```python
from build123d import *

# Parameters (mm, degrees)
F0_W     = 93
F0_H     = 153
F2_DEPTH = 6
F1_W     = 93
F1_H     = 14
F3_DEPTH = 2
F5_D     = 6


with BuildPart() as f2:
    # F0 (on Top) → F2 (new body)
    with BuildSketch(Plane.XY):
        with BuildLine():
            Line((-73.5, -125.5), (73.5, -125.5))
            ThreePointArc((73.5, -125.5), (79.1568542495, -123.1568542495), (81.5, -117.5))
            Line((81.5, -117.5), (81.5, 117.5))
            ThreePointArc((81.5, 117.5), (79.1568542495, 123.1568542495), (73.5, 125.5))
            Line((73.5, 125.5), (-73.5, 125.5))
            ThreePointArc((-73.5, 125.5), (-79.1568542495, 123.1568542495), (-81.5, 117.5))
            Line((-81.5, 117.5), (-81.5, -117.5))
            ThreePointArc((-81.5, -117.5), (-79.1568542495, -123.1568542495), (-73.5, -125.5))
        make_face()
        Rectangle(F0_W, F0_H, mode=Mode.SUBTRACT)
    extrude(amount=-F2_DEPTH)

    # F1 (on face) → F3 (cut)
    with BuildSketch(Plane.XY):
        with Locations((0, 83.5)):
            Rectangle(F1_W, F1_H)
        with Locations((0, -83.5)):
            Rectangle(F1_W, F1_H)
    extrude(amount=-F3_DEPTH, mode=Mode.SUBTRACT)

    # F5 (through all)
    with Locations(Plane.XY):
        with Locations((-37.3, 83), (37.3, 83), (37.3, -83), (-37.3, -83)):
            Hole(F5_D / 2)


solid = f2.part
```
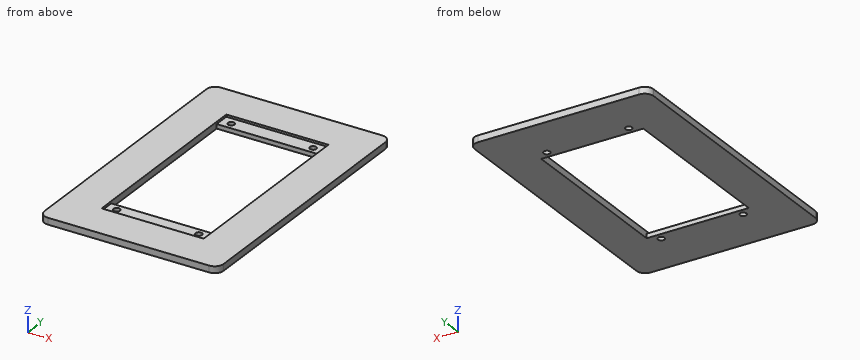
Work out the finished part from the listing and answer in its coordinate system (mm). Coordinates: 2 decimals unless noted, no trailing zeros. Loops run counter-clockwise (first coordinate to the right, second up) from the corner with the lowest first, then second, coordinate; pieces in that order, holes last.
1) Section C-C (y = -83) is taken. Give the vertices of the cut face in (x, z), plus the area to 3 significant figures.
Results:
outline: (-81.5, -6) - (-40.3, -6) - (-40.3, -2) - (-46.5, -2) - (-46.5, 0) - (-81.5, 0) - close; (-34.3, -6) - (34.3, -6) - (34.3, -2) - (-34.3, -2) - close; (40.3, -6) - (81.5, -6) - (81.5, 0) - (46.5, 0) - (46.5, -2) - (40.3, -2) - close
area: 744 mm2
2) A flat-ended cylindrical pin translates along its axis: pin 1 (15.5 mm diameter, centred on x = -16.5, y = -82.5, fed in from +Z). Find the tip coordinate at first contact, or state that the pin passes through.
Results:
pin 1: stops at z = -2
3) Section B-B (z = -4.75) is taken. Give the vertices of the cut face in (x, y).
Results:
outline: (-81.5, -117.5) arc R8 ccw to (-73.5, -125.5) - (73.5, -125.5) arc R8 ccw to (81.5, -117.5) - (81.5, 117.5) arc R8 ccw to (73.5, 125.5) - (-73.5, 125.5) arc R8 ccw to (-81.5, 117.5) - close; hole (-46.5, -76.5) - (46.5, -76.5) - (46.5, 76.5) - (-46.5, 76.5) - close; hole circle Ø6 at (-37.3, -83); hole circle Ø6 at (-37.3, 83); hole circle Ø6 at (37.3, -83); hole circle Ø6 at (37.3, 83)
4) Consider probe 1 along Y at (x, z) = (37.3, -3.25); probe 2 along X at (y, z) = (34.5, -3.6); probe 3 along Y at (x, z) = (19.5, -4.85). Determine where each line is inside the solid, lowest interval first.
Results:
probe 1: y = -125.5 to -86, -80 to -76.5, 76.5 to 80, 86 to 125.5
probe 2: x = -81.5 to -46.5, 46.5 to 81.5
probe 3: y = -125.5 to -76.5, 76.5 to 125.5
5) Section A-A (x = -37.3) is taken. Give the vertices of the cut face in (y, z).
Results:
outline: (-125.5, -6) - (-86, -6) - (-86, -2) - (-90.5, -2) - (-90.5, 0) - (-125.5, 0) - close; (-80, -6) - (-76.5, -6) - (-76.5, -2) - (-80, -2) - close; (76.5, -6) - (80, -6) - (80, -2) - (76.5, -2) - close; (86, -6) - (125.5, -6) - (125.5, 0) - (90.5, 0) - (90.5, -2) - (86, -2) - close
6) Section D-D (x = 31) is taken. Give the vertices of the cut face in (y, z), plus the area to 3 significant figures.
Results:
outline: (-125.5, -6) - (-76.5, -6) - (-76.5, -2) - (-90.5, -2) - (-90.5, 0) - (-125.5, 0) - close; (76.5, -6) - (125.5, -6) - (125.5, 0) - (90.5, 0) - (90.5, -2) - (76.5, -2) - close
area: 532 mm2
